Build history of the part. All positions in model axes, mm. A direction names the side the tool comes from. Give positions to 0.01 mm unless a question says otherwise; leave off trailing zeros. Write each loop counter-clockwise with the first axis right and the second up, starting at its lowest first coordinate (ties: lowest second). Pieces come first, ordered by that corner, then holes. Notation, with made-up numbers: M 16.5,40 L 27.5,40 A36 ccw 27.5,76 Z; hole C 56,23 d3. An arc over 180 degrees is marked long. One line per item, written item: value. Start each with the question number.
from build123d import *

# Parameters (mm, degrees)
SKETCH_1_W      = 50
SKETCH_1_H      = 77
EXTRUDE_1_DEPTH = 3


with BuildPart() as part:
    # 草图1 → 凸台-拉伸1 (new body)
    with BuildSketch(Plane.XY):
        Rectangle(SKETCH_1_W, SKETCH_1_H)
        with BuildLine():
            Line((-12.085786438, 32.25), (-5.75, 32.25))
            Line((-5.75, 32.25), (-5.75, 35.75))
            Line((-5.75, 35.75), (-12.085786438, 35.75))
            ThreePointArc((-12.085786438, 35.75), (-13.5, 36.25), (-14.914213562, 35.75))
            Line((-14.914213562, 35.75), (-21.25, 35.75))
            Line((-21.25, 35.75), (-21.25, 32.25))
            Line((-21.25, 32.25), (-14.914213562, 32.25))
            ThreePointArc((-14.914213562, 32.25), (-13.5, 31.75), (-12.085786438, 32.25))
        make_face(mode=Mode.SUBTRACT)
        with BuildLine():
            Line((21.25, 35.75), (21.25, 32.25))
            Line((21.25, 32.25), (14.914213562, 32.25))
            ThreePointArc((14.914213562, 32.25), (13.5, 31.75), (12.085786438, 32.25))
            Line((12.085786438, 32.25), (5.75, 32.25))
            Line((5.75, 32.25), (5.75, 35.75))
            Line((5.75, 35.75), (12.085786438, 35.75))
            ThreePointArc((12.085786438, 35.75), (13.5, 36.25), (14.914213562, 35.75))
            Line((14.914213562, 35.75), (21.25, 35.75))
        make_face(mode=Mode.SUBTRACT)
        with BuildLine():
            Line((21.25, -35.75), (14.914213562, -35.75))
            ThreePointArc((14.914213562, -35.75), (13.5, -36.25), (12.085786438, -35.75))
            Line((12.085786438, -35.75), (5.75, -35.75))
            Line((5.75, -35.75), (5.75, -32.25))
            Line((5.75, -32.25), (12.085786438, -32.25))
            ThreePointArc((12.085786438, -32.25), (13.5, -31.75), (14.914213562, -32.25))
            Line((14.914213562, -32.25), (21.25, -32.25))
            Line((21.25, -32.25), (21.25, -35.75))
        make_face(mode=Mode.SUBTRACT)
        with BuildLine():
            Line((-21.25, -35.75), (-21.25, -32.25))
            Line((-21.25, -32.25), (-14.914213562, -32.25))
            ThreePointArc((-14.914213562, -32.25), (-13.5, -31.75), (-12.085786438, -32.25))
            Line((-12.085786438, -32.25), (-5.75, -32.25))
            Line((-5.75, -32.25), (-5.75, -35.75))
            Line((-5.75, -35.75), (-12.085786438, -35.75))
            ThreePointArc((-12.085786438, -35.75), (-13.5, -36.25), (-14.914213562, -35.75))
            Line((-14.914213562, -35.75), (-21.25, -35.75))
        make_face(mode=Mode.SUBTRACT)
    extrude(amount=EXTRUDE_1_DEPTH)


solid = part.part
1) Mould opens along X. For faces 3 (the face through (0, -38.5, 1)), 4 (the face through (9, 35.75, 1)), 5 (the face through (21.25, -34, 1)) say: released by +X, released by -X, zero draft, split by the parting line, or undercut.
2) Drop a flat-ended pin along its axis: P1, Ø3, axis at x = -14, y = -28, coming from the -Z side. Give the stop position or say it passes through.
3) Tool access for faces 1 (the face through (-18, 32.25, 1)), 2 (the face through (0, 1, 3)): list every direction of +Z, -Z, +X, -X, +Y, -Y with a clear straight run to the whole face (end or side of a thin tool).
4) Band-saw the part on A-A (x = 7.5). List the corners of the cut face in (y, z), then the cut area to 3 significant figures.
5) Band-saw the part on B-B (z = 2). Count the separate pieces of the cut face and the enclosed holes in it, then the cut area to 3 significant figures.
6) Probe line 1 along Y through (x, z) = (18, 2.8). List the from-to ranges inside material, lowest first. Write a range as from..to.
Model answer:
1. face 3: zero draft
1. face 4: undercut
1. face 5: undercut
2. P1: stops at z = 0
3. face 1: +Z, -Z
3. face 2: +Z, +X, -X, +Y, -Y
4. outline: M -38.5,0 L -35.75,0 L -35.75,3 L -38.5,3 Z; M -32.25,0 L 32.25,0 L 32.25,3 L -32.25,3 Z; M 35.75,0 L 38.5,0 L 38.5,3 L 35.75,3 Z
4. area: 210 mm²
5. separate pieces: 1
5. enclosed holes: 4
5. area: 3,630 mm²
6. line 1: y = -38.5..-35.75, -32.25..32.25, 35.75..38.5
